from build123d import *

# Parameters (mm, degrees)
CUT_EXTRUDE2_DEPTH      = 20.413875706
CUT_EXTRUDE2_DEPTH_BACK = 20.413875706
SKETCH2_W               = 1.17
SKETCH2_H               = 0.79


with BuildPart() as part:
    # Sketch1 → Revolve1 (revolve)
    with BuildSketch(Plane(origin=(0, 0, 0), x_dir=(1, 0, 0), z_dir=(0, 1, 0))):
        with BuildLine():
            Line((0, 0), (2.645379929, 0))
            Line((2.645379929, 0), (2.645379929, 9.53))
            Line((2.645379929, 9.53), (1.8, 9.53))
            Line((1.8, 9.53), (1.8, 17.25))
            ThreePointArc((1.8, 17.25), (1.272792206, 18.522792206), (0, 19.05))
            Line((0, 19.05), (0, 0))
        make_face()
    revolve(axis=Axis((0, 0, 0), (0, 0, -1)))

    # Sketch2 → Cut-Extrude2 (cut, two sides: drawn at the far end of the back side and taken through both)
    with BuildSketch(Plane(origin=(0, 0, 0), x_dir=(1, 0, 0), z_dir=(0, 1, 0)).offset(-CUT_EXTRUDE2_DEPTH_BACK)):
        with Locations((0, 0.395)):
            Rectangle(SKETCH2_W, SKETCH2_H)
    extrude(amount=CUT_EXTRUDE2_DEPTH + CUT_EXTRUDE2_DEPTH_BACK, mode=Mode.SUBTRACT)


solid = part.part
Work out the finished part from the listing and answer in its coordinate system (mm). A direction names the side the tool comes from. Coordinates: 2 decimals unless noted, no trailing zeros. Write each loop counter-clockwise with the first axis right and the second up, starting at its lowest first coordinate (ties: lowest second). Pieces come first, ordered by that corner, then holes.
1. The part is cut by section C-C, the plane z = -4.75. Write down the section's boundary in (x, y).
Results list:
outline: circle Ø5.29 at (0, 0)
2. The part is cut by section A-A, the plane y = 0. Write down the section's boundary in (x, z) (3 decimals), and give its area (3 significant figures).
Results list:
outline: (-2.645, -9.53) - (-1.8, -9.53) - (-1.8, -17.25) arc R1.8 ccw to (1.8, -17.25) - (1.8, -9.53) - (2.645, -9.53) - (2.645, 0) - (0.585, 0) - (0.585, -0.79) - (-0.585, -0.79) - (-0.585, 0) - (-2.645, 0) - close
area: 82.4 mm2
3. Flat-ended cylindrical pins translate along their axes: pin 1 (1.6 mm diameter, centred on x = 0, y = 1, fed in from -Z); pin 2 (0.9 mm diameter, centred on x = 0, y = -0.5, fed in from +Z); pin 3 (2 mm diameter, centred on x = 0, z = -12, fed in from +Y). Find the tip coordinate at first contact, or state that the pin passes through.
Results list:
pin 1: stops at z = -19.04
pin 2: stops at z = -0.79
pin 3: stops at y = 1.8
4. For a pull along X with two mould halves and no side action, classify faces 3 (the cylindrical face through (1.717, -0.541, -13.444)), 4 (the flat face through (0, 0, -0.79)), 5 (the flat face through (1, 0, 0)) as +X half, -X half, draft (parallel to the pull), parting line (faces both ways), or undercut.
Results list:
face 3: parting line
face 4: undercut
face 5: draft
5. The part is cut by section B-B, the plane x = 0. Write down the section's boundary in (y, z).
Results list:
outline: (-2.65, -9.53) - (-1.8, -9.53) - (-1.8, -17.25) arc R1.8 ccw to (1.8, -17.25) - (1.8, -9.53) - (2.65, -9.53) - (2.65, -0.79) - (-2.65, -0.79) - close
6. For faces 1 (the flat face through (1, 2, -9.53)), 2 (the flat face through (-1, 0, 0)), determine the directions among +Z, -Z, +X, -X, +Y, -Y from which every point of the face is accessible in a straight line to the end or side of a thin tool.
Results list:
face 1: -Z
face 2: +Z, +X, -X, +Y, -Y
7. The part is cut by section D-D, the plane y = -1.4. Write down the section's boundary in (x, z) (3 decimals).
Results list:
outline: (-2.245, -9.53) - (-1.131, -9.53) - (-1.131, -17.25) arc R1.131 ccw to (1.131, -17.25) - (1.131, -9.53) - (2.245, -9.53) - (2.245, 0) - (0.585, 0) - (0.585, -0.79) - (-0.585, -0.79) - (-0.585, 0) - (-2.245, 0) - close
8. Consider line 1 along Z through (x, y) = (2.25, 0.5); line 2 along Y through (x, z) = (0.25, -1.75); line 3 along X through (y, z) = (1.4, -5.75). Determine where each line is inside the solid, lowest interval first.
Results list:
line 1: z = -9.53 to 0
line 2: y = -2.63 to 2.63
line 3: x = -2.24 to 2.24
